Work out the finished part from the listing and answer in its coordinate system (mm). A direction names the side the tool comes from. Coordinates: 2 decimals unless noted, no trailing zeros. Order: outer loops, then holes, each group sorted by start corner. A loop starts at its lowest first (then second) coordinate and runs counter-clockwise, first axis right, second up. Notation, with made-up numbers: (61.5, 82.5) -> (100.5, 82.5) arc R25 ccw to (100.5, 119.5) -> close; hole circle Ø6 at (61, 19). An arc over 180 degrees is marked (long way). Use one line per item in the form item = value.
from build123d import *

# Parameters (mm, degrees)
F0_W     = 44.3
F0_H     = 53.5
F1_DEPTH = 21.3
F2_R     = 11.39
F3_R     = 11.391
F4_R     = 11.391
F5_R     = 9.3
F6_W     = 6.7
F6_H     = 1.5
F7_DEPTH = 6.7


with BuildPart() as f1:
    # F0 (on Front) → F1 (new body)
    with BuildSketch(Plane.XZ):
        with Locations((22.15, 26.75)):
            Rectangle(F0_W, F0_H)
    extrude(amount=F1_DEPTH)

    # F2
    f2_edges = [f1.edges().sort_by_distance(p)[0] for p in [
        (44.3, -10.65, 0),
    ]]
    fillet(f2_edges, radius=F2_R)

    # F3
    f3_edges = [f1.edges().sort_by_distance(p)[0] for p in [
        (0, -10.65, 0),
    ]]
    fillet(f3_edges, radius=F3_R)

    # F4
    f4_edges = [f1.edges().sort_by_distance(p)[0] for p in [
        (44.3, -10.65, 53.5),
        (0, -10.65, 53.5),
    ]]
    fillet(f4_edges, radius=F4_R)

    # F5
    f5_edges = [f1.edges().sort_by_distance(p)[0] for p in [
        (3.336347, -21.3, 50.163653),
        (3.336347, 0, 50.163653),
    ]]
    fillet(f5_edges, radius=F5_R)

    # F6 (on face) → F7 (cut)
    with BuildSketch(Plane(origin=(0, 0, 0), x_dir=(1, 0, 0), z_dir=(0, 0, -1))):
        with Locations((22.15018, 10.65)):
            Rectangle(F6_W, F6_H)
    extrude(amount=-F7_DEPTH, mode=Mode.SUBTRACT)


solid = f1.part
(1) Each of these flat-tipped pins is pushed along its axis until it touches: P1, Ø1, axis at y = -12.5, z = 10.5, coming from the +X side; P2, Ø3.5, axis at x = 21.5, z = 4, coming from the +Y side; P3, Ø5.5, axis at x = 22, z = 3, coming from the -Y side. Where does it stop, or does it pass through?
Data:
P1 = 44.29
P2 = -0.7
P3 = -20.6
(2) Section A-A on x = 24.5 is taken. Write down the section's boundary in (y, z), plus the area to 3 significant figures.
Data:
outline = (-21.3, 9.3) arc R9.3 ccw to (-12, 0) -> (-11.4, 0) -> (-11.4, 6.7) -> (-9.9, 6.7) -> (-9.9, 0) -> (-9.3, 0) arc R9.3 ccw to (0, 9.3) -> (0, 44.2) arc R9.3 ccw to (-9.3, 53.5) -> (-12, 53.5) arc R9.3 ccw to (-21.3, 44.2) -> close
area = 1,060 mm²
(3) The mould has two halves that part along X. Classify faces 1 (the flat face through (22, -11, 53.5)), 2 (the cylindrical face through (41.5, -2.65, 26.53)), 3 (the flat face through (18.8, -11, 3)): released by +X, released by -X, zero draft, split by the parting line, or undercut.
Data:
face_1 = zero draft
face_2 = released by +X
face_3 = undercut
(4) Straight lines are drawn through the part: line 1 along Z through (x, y) = (24.5, -16.5); line 2 along Z through (x, y) = (21, -16.75); line 3 along Y through (x, z) = (38, 19.5). For each, find the intervals that lie inside material, in ascending order.
Data:
line_1 = 1.16 to 52.34
line_2 = 1.3 to 52.2
line_3 = -20.8 to -0.5
(5) Section B-B on z = 31.5 is taken. Write down the section's boundary in (x, y), plus the area to 3 significant figures.
Data:
outline = (0, -12) arc R9.3 ccw to (9.3, -21.3) -> (35, -21.3) arc R9.3 ccw to (44.3, -12) -> (44.3, -9.3) arc R9.3 ccw to (35, 0) -> (9.3, 0) arc R9.3 ccw to (0, -9.3) -> close
area = 869 mm²
(6) Which of the six approach directions +Z, -Z, +X, -X, +Y, -Y give full straight-line access (tool end or side, diameter ignored) to faces 4 (the cylindrical face through (22, -2.65, 2.8)), 5 (the flat face through (22, -11, 6.7))?
Data:
face_4 = -Z, +X, -X, +Y
face_5 = -Z
